```python
from build123d import *

# Parameters (mm, degrees)
SKETCH_R        = 2
SKETCH_R_2      = 11.5
SKETCH_R_3      = 1.6
SKETCH_R_4      = 1.5
PAD_DEPTH       = 28
SKETCH003_W     = 29
SKETCH003_H     = 20
POCKET_DEPTH    = 42
SKETCH004_R     = 3
POCKET001_DEPTH = 26
SKETCH005_R     = 3
POCKET002_DEPTH = 42
SKETCH006_W     = 16
SKETCH006_H     = 20
POCKET003_DEPTH = 16
SKETCH007_W     = 27
SKETCH007_H     = 20
POCKET004_DEPTH = 10


with BuildPart() as part:
    # Sketch → Pad (new body)
    with BuildSketch(Plane.XY):
        Polygon((-17, 21), (-21, 17), (-21, -17), (-17, -21), (42, -21), (44, -19), (44, -5), (42, -3), (23, -3), (21, -1), (21, 17), (17, 21), align=None)
        with Locations((-15.5, -15.5)):
            Circle(SKETCH_R, mode=Mode.SUBTRACT)
        with Locations((15.5, -15.5)):
            Circle(SKETCH_R, mode=Mode.SUBTRACT)
        with Locations((15.5, 15.5)):
            Circle(SKETCH_R, mode=Mode.SUBTRACT)
        with Locations((-15.5, 15.5)):
            Circle(SKETCH_R, mode=Mode.SUBTRACT)
        Circle(SKETCH_R_2, mode=Mode.SUBTRACT)
        with Locations((28, -11)):
            Circle(SKETCH_R_3, mode=Mode.SUBTRACT)
        with Locations((39, -11)):
            Circle(SKETCH_R_4, mode=Mode.SUBTRACT)
    extrude(amount=PAD_DEPTH)

    # Sketch003 (on Face4 of Pad) → Pocket (cut)
    with BuildSketch(Plane.XZ.offset(21)):
        with Locations((35.5, 14)):
            Rectangle(SKETCH003_W, SKETCH003_H)
    extrude(amount=-POCKET_DEPTH, mode=Mode.SUBTRACT)

    # Sketch004 (on Face5 of Pocket) → Pocket001 (cut)
    with BuildSketch(Plane.XY.offset(28)):
        with Locations((-15.5, -15.5)):
            Circle(SKETCH004_R)
        with Locations((-15.5, 15.5)):
            Circle(SKETCH004_R)
        with Locations((15.5, 15.5)):
            Circle(SKETCH004_R)
        with Locations((15.5, -15.5)):
            Circle(SKETCH004_R)
    extrude(amount=-POCKET001_DEPTH, mode=Mode.SUBTRACT)

    # Sketch005 (on Face14 of Pocket001) → Pocket002 (cut)
    with BuildSketch(Plane.YZ.offset(21)):
        with Locations((-11, 14)):
            Circle(SKETCH005_R)
    extrude(amount=-POCKET002_DEPTH, mode=Mode.SUBTRACT)

    # Sketch006 (on Face15 of Pocket002) → Pocket003 (cut)
    with BuildSketch(Plane.YZ.offset(21)):
        with Locations((2, 14)):
            Rectangle(SKETCH006_W, SKETCH006_H)
    extrude(amount=-POCKET003_DEPTH, mode=Mode.SUBTRACT)

    # Sketch007 (on Face36 of Pocket003) → Pocket004 (cut)
    with BuildSketch(Plane(origin=(0, -6, 0), x_dir=(-1, 0, 0), z_dir=(0, 1, 0))):
        with Locations((-4.5, 14.038037)):
            Rectangle(SKETCH007_W, SKETCH007_H)
    extrude(amount=-POCKET004_DEPTH, mode=Mode.SUBTRACT)


solid = part.part
```
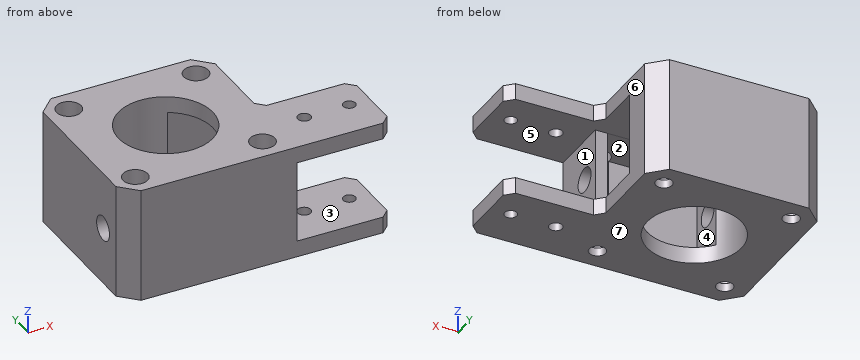
Source: CAD feature listing. Evaluate the final solid. Frame: model axes, mm. Face numbers are marked on the shaded views. A direction names the side the tool comes from. Round coordinates to 2 decimals unless told otherwise and drop trailing zeros. Loops run counter-clockwise (first coordinate to the right, second up) from the corner with the lowest first, then second, coordinate; pieces in that order, holes last.
1. Section query D-D on z = 25.75. Output: boundary loops of the cut face in (x, y), and give its area (3 significant figures).
2. Mould query, pull axis Z, two halves, no side actions, for the marked faces 4, 5, 6 and 7. Classes: released by +Z, released by -Z, zero draft, split by the parting line, or undercut.
3. Access query for the marked faces 1, 2 and 3. Directions: +Z, -Z, +X, -X, +Y, -Y. A direction counts if a zero-diameter tool reaches every point of the face in a straight line with its end or side. Return the directions, or none.
4. Contact query for flat-ended pins moving along their axis: pin 1 (9.5 mm diameter, centred on y = -10, z = 13.5, fed in from +X); pin 2 (1.8 mm diameter, centred on x = -15.5, y = -14, fed in from +Z); pin 3 (8 mm diameter, centred on x = 6.5, y = -10, fed in from -Z). Output: stop coordinate, or through.
5. Section query B-B on x = 15.5. Give the number of separate pieces and of enclosed holes in the cut face, and give its area (3 significant figures).
6. Section query A-A on x = 28. Output: boundary loops of the cut face in (y, z).
7. Section query C-C on y = 7. Output: boundary loops of the cut face in (x, z).
8. Ray query, L1, parallel to Y at x = 15.5, z = 18.25; L2, parallel to Y at x = -15.5, z = 1.5; L3, parallel to Y at x = 20.5, z = 20.75. Return the intervals inside material, ascending.
Answers below:
1. outline: (-21, -17) - (-17, -21) - (42, -21) - (44, -19) - (44, -5) - (42, -3) - (23, -3) - (21, -1) - (21, 17) - (17, 21) - (-17, 21) - (-21, 17) - close; hole circle Ø6 at (-15.5, -15.5); hole circle Ø6 at (-15.5, 15.5); hole circle Ø23 at (0, 0); hole circle Ø6 at (15.5, -15.5); hole circle Ø6 at (15.5, 15.5); hole circle Ø3.2 at (28, -11); hole circle Ø3 at (39, -11)
1. area: 1,610 mm2
2. face 4: undercut
2. face 5: undercut
2. face 6: zero draft
2. face 7: released by -Z
3. face 1: +X, +Y, -Y
3. face 2: none
3. face 3: +X
4. pin 1: stops at x = 21
4. pin 2: stops at z = 2
4. pin 3: stops at z = 0
5. separate pieces: 3
5. enclosed holes: 0
5. area: 398 mm2
6. outline: (-21, 0) - (-12.6, 0) - (-12.6, 4) - (-21, 4) - close; (-21, 24) - (-12.6, 24) - (-12.6, 28) - (-21, 28) - close; (-9.4, 0) - (-3, 0) - (-3, 4) - (-9.4, 4) - close; (-9.4, 24) - (-3, 24) - (-3, 28) - (-9.4, 28) - close
7. outline: (-21, 0) - (-9.12, 0) - (-9.12, 28) - (-21, 28) - close; (9.12, 0) - (21, 0) - (21, 4) - (9.12, 4) - close; (9.12, 24) - (21, 24) - (21, 28) - (9.12, 28) - close
8. L1: y = -21 to -18.5, 10 to 12.5, 18.5 to 21
8. L2: y = -21 to -17.5, -13.5 to 13.5, 17.5 to 21
8. L3: y = -21 to -6, 10 to 17.5
